Autodesk Inventor part; units mm, degrees
ref_plane "Work Plane2" through (-6.985, 321.137, 5.08) normal (0, 0, -1) x (0, 1, 0)
ref_plane "YZ Plane" through (0, 0, 0) normal (1, 0, 0) x (0, 1, 0)
ref_plane "XZ Plane" through (0, 0, 0) normal (0, 1, 0) x (-1, 0, 0)
ref_plane "Work Plane1" through (0, 0, 0) normal (0, 0, 1) x (1, 0, 0)
sketch "Sketch1" plane through (0, 0, 0) normal (0, 0, 1) x (1, 0, 0)
  line L0 (12.9032, 330.789) -> (12.9032, 321.137)
  line L1 (-6.985, 321.137) -> (-6.985, 330.0524)
  line L2 (3.1132, 307.8274) -> (-3.1132, 307.8274)
  line L3 (3.1132, 340.8474) -> (-3.1132, 340.8474)
  line L4 (12.9032, 340.8474) -> (-6.985, 340.8474)
  line L5 (-6.985, 340.8474) -> (-6.985, 307.8274)
  line L6 (-6.985, 307.8274) -> (12.9032, 307.8274)
  line L7 (12.9032, 307.8274) -> (12.9032, 340.8474)
  arc A0 (-1.7468, 337.6651) -> (-1.3298, 338.9494) centre (0, 337.8078) ccw
  arc A1 (-1.7468, 310.7243) -> (-1.3298, 312.0086) centre (0, 310.867) ccw
  circle A2 centre (0, 337.8078) radius 1.778
  point P0 (0, 0)
  dimension "d2" = 3.556
ref_plane "Work Plane2" through (-6.985, 321.137, 5.08) normal (0, 0, -1) x (0, 1, 0)
extrude "Extrusion1" add sketch "Sketch1" along normal up to surface (5.08 mm away) contours L0 L7 L6 L2 L5 L1 L4 L3 | A2
sketch "Sketch3" plane through (-6.985, 340.8474, 5.08) normal (0, 0, 1) x (1, 0, 0)
  circle A0 centre (5.1816, -17.2783) radius 1.1938
  circle A1 centre (14.7066, -17.2783) radius 1.1938
  circle A2 centre (5.1816, -17.2783) radius 1.1938
  circle A3 centre (14.7066, -17.2783) radius 1.1938
  arc A4 (8.2018, -4.301) -> (6.9677, -4.7921) centre (6.985, -3.0396) ccw
  arc A5 (8.2018, -31.2417) -> (6.9677, -31.7329) centre (6.985, -29.9804) ccw
  circle A6 centre (6.985, -3.0396) radius 1.778
  circle A7 centre (6.985, -29.9804) radius 1.778
  arc A8 (8.2018, -31.2417) -> (6.9677, -31.7329) centre (6.985, -29.9804) ccw
  circle A9 centre (6.985, -29.9804) radius 1.778
  point P0 (6.985, -340.8474)
  dimension "d17" = 3.556
  dimension "d18" = 3.556
  dimension "d26" = 3.556
sketch "Sketch4" plane through (0, 0, 0) normal (0, 0, -1) x (-1, 0, 0)
  circle A0 centre (1.8034, 323.5691) radius 1.1938
  circle A1 centre (-7.7216, 323.5691) radius 1.1938
  circle A2 centre (1.8034, 323.5691) radius 1.1938
  circle A3 centre (-7.7216, 323.5691) radius 1.1938
  point P0 (0, 0)
hole "Hole1" at (-1.8034, 323.5691, 0) direction (0, 0, 1) diameter 2.3876 end through all counterbore diameter 5.08 counterbore depth 1.905
sketch "Sketch5" plane through (0, 0, 0) normal (0, 0, -1) x (-1, 0, 0)
  circle A0 centre (-7.7216, 323.5691) radius 1.1938
  circle A1 centre (-7.7216, 323.5691) radius 1.1938
  circle A2 centre (-7.7216, 323.5691) radius 1.1938
  point P0 (0, 0)
hole "Hole2" at (7.7216, 323.5691, 0) direction (0, 0, 1) diameter 2.3876 end through all counterbore diameter 5.08 counterbore depth 1.905
hole "Hole3" at (0, 337.8078, 5.08) direction (0, 0, -1) diameter 3.556 end through all
sketch "Sketch6" plane through (0, 0, 0) normal (0, 0, -1) x (-1, 0, 0)
  arc A0 (0.0173, 309.1145) -> (-1.2168, 309.6057) centre (0, 310.867) ccw
  circle A1 centre (0, 310.867) radius 1.778
  point P0 (0, 0)
  dimension "d27" = 3.556
hole "Hole4" at (0, 310.867, 0) direction (0, 0, 1) diameter 3.556 end through all
fillet "Fillet1" radius 3.175 1 edges at (-6.985, 307.8274, 2.54)
fillet "Fillet2" radius 3.175 1 edges at (-6.985, 340.8474, 2.54)
fillet "Fillet3" radius 3.175 1 edges at (12.9032, 307.8274, 2.54)
fillet "Fillet4" radius 3.175 1 edges at (12.9032, 340.8474, 2.54)
properties part number "Switch on T nut holder"
Design review of the part built by this model. Coordinates are the model's own, in mm. A direction names the side the tool comes from. Give positions to 0.01 mm unless a question says otherwise; leave off trailing zeros. Order: outer loops, then holes, each group sorted by start corner. A loop starts at its lowest first (then second) coordinate and runs counter-clockwise, first axis right, second up. Notation, with made-up numbers: (20.25, 15.5) -> (31.25, 15.5) arc R22 cw to (31.25, 23.5) -> close; hole circle Ø5 at (85.25, 58). An arc over 180 degrees is marked (long way). Write item = value, one per line. Start each with the question number.
(1) We need section A-A on y = 323. Write out the cut boundary in (x, z) (3 decimals).
(2) Mouldability with a two-part tool opening along X and no side actions: class faces 1 (the face through (-0.534, 312.563, 2.576)), 2 (the face through (3, 325, 0)), 3 (the face through (11.948, 308.733, 2.576)), 4 (the face through (7.669, 322.376, 3.515)) as +X half, -X half, draft (parallel to the pull), parting line (faces both ways), or undercut.
(3) To check wall thickness, follow line 1 along X through (y, z) = (310, 3.85); line 2 along X through (y, z) = (339, 1.1); line 3 along X through (y, z) = (324, 1.2) (3 decimals). State the ranges of each line that lie inside material, in increasing order.
(4) We need section B-B on x = 0. Write out the cut boundary in (y, z) (3 decimals).
(5) For faces 5 (the face through (9, 324, 1.905)), 6 (the face through (-0.078, 339.584, 2.504)), list the 3-axis set-ups (+Z, -Z, +X, -X, +Y, -Y) from which the entire face can be reached by the end or side of a thin tool; tool diameter is ignored.
(6) For pin 1 (6 mm diameter, centred on x = 7.72, y = 323.57, fed in from +Z); pin 2 (4.5 mm diameter, centred on x = -1.8, y = 323.57, fed in from -Z) (3 decimals), all flat-tipped, find the tip position at first contact; note any pin that passes through.
(7) We need section D-D on z = 4.05. Write out the cut boundary in (x, y) (3 decimals).
(8) We need section C-C on y = 338.5. Write out the cut boundary in (x, z).
Numbers:
q1.outline = (-6.985, 0) -> (-4.279, 0) -> (-4.279, 1.905) -> (-2.853, 1.905) -> (-2.853, 5.08) -> (-6.985, 5.08) -> close; (-0.754, 1.905) -> (0.672, 1.905) -> (0.672, 0) -> (5.246, 0) -> (5.246, 1.905) -> (6.672, 1.905) -> (6.672, 5.08) -> (-0.754, 5.08) -> close; (8.771, 1.905) -> (10.197, 1.905) -> (10.197, 0) -> (12.903, 0) -> (12.903, 5.08) -> (8.771, 5.08) -> close
q2.face_1 = undercut
q2.face_2 = draft
q2.face_3 = +X half
q2.face_4 = undercut
q3.line_1 = -6.82 to -1.55, 1.55 to 12.74
q3.line_2 = -6.69 to -1.32, 1.32 to 12.61
q3.line_3 = -6.985 to -4.307, 0.7 to 5.218, 10.225 to 12.903
q4.outline = (307.827, 0) -> (309.089, 0) -> (309.089, 5.08) -> (307.827, 5.08) -> close; (312.645, 0) -> (321.78, 0) -> (321.78, 1.905) -> (325.358, 1.905) -> (325.358, 0) -> (336.03, 0) -> (336.03, 5.08) -> (312.645, 5.08) -> close; (339.586, 0) -> (340.847, 0) -> (340.847, 5.08) -> (339.586, 5.08) -> close
q5.face_5 = -Z
q5.face_6 = +Z, -Z
q6.pin_1 = 5.08
q6.pin_2 = 1.905
q7.outline = (-6.985, 311.002) arc R3.175 ccw to (-3.81, 307.827) -> (9.728, 307.827) arc R3.175 ccw to (12.903, 311.002) -> (12.903, 337.672) arc R3.175 ccw to (9.728, 340.847) -> (-3.81, 340.847) arc R3.175 ccw to (-6.985, 337.672) -> close; hole circle Ø2.388 at (-1.803, 323.569); hole circle Ø3.556 at (0, 310.867); hole circle Ø3.556 at (0, 337.808); hole circle Ø2.388 at (7.722, 323.569)
q8.outline = (-6.88, 0) -> (-1.64, 0) -> (-1.64, 5.08) -> (-6.88, 5.08) -> close; (1.64, 0) -> (12.79, 0) -> (12.79, 5.08) -> (1.64, 5.08) -> close
